Check sheet for the modelled part. Datum: model origin and axes. Units: mm. A direction names the side the tool comes from. Round coordinates to 2 decimals unless told otherwise and drop trailing zeros. Loops run counter-clockwise (first coordinate to the right, second up) from the corner with the lowest first, then second, coordinate; pieces in that order, holes last. Notation, with made-up numbers: (-26, -22.5) - (29, -22.5) arc R29 cw to (29, 5.5) - close; hole circle Ø8 at (74, 59.5). An arc over 180 degrees is marked (long way). Answer in a Markdown table with one row per item. Add a question column.
(1) Cross-section at D-D on y = 0. Enter the section's corners in (x, z).
(2) Gauge pin test, flat ends, axial feed: pin 1 (4.5 mm diameter, centred on y = -8.5, z = 7, fed in from -X); pin 2 (2 mm diameter, centred on y = 2.5, z = 9.5, fed in from +X); pin 3 (6 mm diameter, centred on y = -14.5, z = 7.5, fed in from +X); pin 4 (1.2 mm diameter, centred on x = -6.85, z = 8, fed in from -Y). Record the tip position at first contact, or that the pin passes through.
(3) Mould release check, pull along Y, two halves, no side actions. Record for faces 4 (the cylindrical face through (15.36, -19.19, 8.13)), 5 (the flat face through (0, 10, 3)), 6 (the cylindrical face through (4.608, 0.361, 4.056)): +Y half, -Y half, draft (parallel to the pull), parting line (faces both ways), or undercut.
(4) Cross-section at C-C on z = 3.25. Enter the section's corners in (x, y).
(5) Cross-section at B-B on x = -27.5. Enter the section's corners in (y, z), then the cut area to 3 significant figures.
(6) Access from +Z, -Z, +X, -X, +Y, -Y to the whole of each face (thin tool, end or side, straight path). Record for faces 1 (the flat face through (-5.5, 7, 6)), 2 (the flat face through (-21.6, -15, 6)), 3 (the flat face through (5.5, -8, 6)).
(7) Thickness scan on line 1 along Y through (x, z) = (-2, 5.25); line 2 along X through (y, z) = (-19.15, 8); line 3 along X through (y, z) = (-17.25, 2.75). Record the ranges inside material, lowest first.
(8) Cross-section at A-A on y = -17.75. Enter the section's corners in (x, z), then the cut area to 3 significant figures.
Autodesk Inventor part; units mm, degrees
ref_plane "YZ Plane" through (0, 0, 0) normal (1, 0, 0) x (0, 1, 0)
ref_plane "XZ Plane" through (0, 0, 0) normal (0, 1, 0) x (-1, 0, 0)
ref_plane "XY Plane" through (0, 0, 0) normal (0, 0, 1) x (1, 0, 0)
sketch "Эскиз1" plane through (0, 0, 0) normal (0, 0, 1) x (1, 0, 0)
  line L0 (-24, 10) -> (24, 10)
  line L1 (24, 10) -> (24, -10) construction
  line L2 (24, -10) -> (-24, -10)
  line L3 (-24, -10) -> (-24, 10) construction
  line L4 (0, 10) -> (0, -10)
  arc A0 (-30.4971, 2.649) -> (-30.4971, -2.649) centre (-27.5, 0) ccw
  line L5 (-30.4971, 2.649) -> (-24, 10)
  line L6 (-30.4971, -2.649) -> (-24, -10)
  arc A1 (30.4971, -2.649) -> (30.4971, 2.649) centre (27.5, 0) ccw
  line L7 (30.4971, 2.649) -> (24, 10)
  line L8 (30.4971, -2.649) -> (24, -10)
  point P0 (0, 0)
  point P1 (0, 0)
  dimension "d0" = 20
  dimension "d1" = 48
  dimension "d2" = 4
  dimension "d3" = 55
extrude "Выдавливание1" add sketch "Эскиз1" along normal blind 2
sketch "Эскиз2" plane through (0, 0, 2) normal (0, 0, 1) x (1, 0, 0)
  line L0 (24, 10) -> (-24, 10)
  line L1 (24, -10) -> (30.4971, -2.649)
  line L2 (-24, 10) -> (24, 10)
  line L3 (24, 10) -> (24, -10)
  line L4 (24, -10) -> (-24, -10)
  line L5 (-24, -10) -> (-24, 10)
  point P0 (0, 0)
extrude "Выдавливание2" add sketch "Эскиз2" along normal blind 6
sketch "Эскиз3" plane through (0, 0, 8) normal (0, 0, 1) x (1, 0, 0)
  circle A0 centre (-12.8, 0) radius 8.2
  circle A1 centre (12.8, 0) radius 8.2
  line L0 (-24, -10) -> (24, -10)
  line L1 (0, -10) -> (0, 10)
  line L2 (24, 10) -> (-24, 10)
  point P0 (0, 0)
  dimension "d8" = 25.6
  dimension "d9" = 16.4
extrude "Выдавливание3" cut sketch "Эскиз3" against normal through all
sketch "Эскиз4" plane through (0, 0, 8) normal (0, 0, 1) x (1, 0, 0)
  line L0 (24, 10) -> (-24, 10)
  line L1 (-5.5, 10) -> (5.5, 10)
  line L2 (5.5, 10) -> (5.5, 5)
  line L3 (5.5, 5) -> (-5.5, 5)
  line L4 (-5.5, 5) -> (-5.5, 10)
  line L5 (-24, 10) -> (-24, -10) construction
  line L6 (-24, 0) -> (24, 0)
  line L7 (24, -10) -> (24, 10) construction
  line L8 (-5.5, -10) -> (5.5, -10)
  line L9 (5.5, -10) -> (5.5, -5)
  line L10 (5.5, -5) -> (-5.5, -5)
  line L11 (-5.5, -5) -> (-5.5, -10)
  point P0 (0, 0)
  point P1 (0, 0)
  point P2 (0, 5)
  point P3 (0, -5)
  dimension "d12" = 5
  dimension "d13" = 11
extrude "Выдавливание4" cut sketch "Эскиз4" against normal blind 4
sketch "Эскиз5" plane through (0, 0, 2) normal (0, 0, 1) x (1, 0, 0)
  arc A0 (-30.4971, 2.649) -> (-30.4971, -2.649) centre (-27.5, 0) ccw
  arc A1 (30.4971, -2.649) -> (30.4971, 2.649) centre (27.5, 0) ccw
  point P0 (0, 0)
  point P1 (27.5, 0)
hole "Отверстие1" at (-27.5, 0, 2) at (27.5, 0, 2) direction (0, 0, -1) diameter 2.8 end through all
sketch "Эскиз6" plane through (0, 0, 0) normal (0, 0, -1) x (-1, 0, 0)
  line L0 (24, -10) -> (-24, -10)
  line L1 (24, -10) -> (-24, -10)
  line L2 (-24, -10) -> (-24, -20)
  line L3 (-24, -20) -> (24, -20)
  line L4 (24, -20) -> (24, -10)
  line L5 (-5.5, -10) -> (5.5, -10)
  line L6 (0, -20) -> (0, -10)
  line L7 (21.6, -18.4) -> (1.6, -18.4)
  line L8 (1.6, -18.4) -> (1.6, -11.4)
  line L9 (1.6, -11.4) -> (21.6, -11.4)
  line L10 (21.6, -11.4) -> (21.6, -18.4)
  line L11 (-1.6, -11.4) -> (-21.6, -11.4)
  line L12 (-21.6, -11.4) -> (-21.6, -18.4)
  line L13 (-21.6, -18.4) -> (-1.6, -18.4)
  line L14 (-1.6, -18.4) -> (-1.6, -11.4)
  point P0 (0, 0)
  point P1 (0, -10)
  dimension "d25" = 10
  dimension "d26" = 48
  dimension "d41" = 20
  dimension "d42" = 7
  dimension "d43" = 1.6
  dimension "d44" = 3.2
extrude "Выдавливание5" add sketch "Эскиз6" against normal blind 12
sketch "Эскиз7" plane through (-24, -20, 0) normal (0, -1, 0) x (1, 0, 0)
  line L0 (24, 0) -> (24, 12)
  line L1 (48, 0) -> (0, 0)
  line L2 (48, 0) -> (0, 0)
  line L3 (48, 0) -> (48, 12)
  line L4 (0, 12) -> (48, 12)
  line L5 (0, 0) -> (0, 12)
  line L6 (45.6, 0) -> (25.6, 0)
  line L7 (45.6, 0) -> (45.6, 12)
  line L8 (25.6, 12) -> (45.6, 12)
  line L9 (25.6, 0) -> (25.6, 12)
  line L10 (22.4, 0) -> (2.4, 0)
  line L11 (22.4, 0) -> (22.4, 12)
  line L12 (2.4, 12) -> (22.4, 12)
  line L13 (2.4, 0) -> (2.4, 12)
  line L14 (0, 12) -> (48, 12)
  line L15 (12.4, 12) -> (12.4, 0)
  line L16 (45, 0) -> (28.6, 0)
  line L17 (35.6, 0) -> (35.6, 12)
  point P0 (7.65, 8)
  point P1 (17.15, 8)
  point P2 (30.85, 8)
  point P3 (40.35, 8)
  dimension "d46" = 9.5
  dimension "d47" = 8
hole "Отверстие2" at (-16.35, -20, 8) at (-6.85, -20, 8) at (6.85, -20, 8) at (16.35, -20, 8) direction (0, 1, 0) diameter 2 depth 11
properties part number "FrontSensor"
Answers:
| question | item | result |
|---|---|---|
| 1 | outline | (-31.5, 0) - (-28.9, 0) - (-28.9, 2) - (-31.5, 2) - close; (-26.1, 0) - (-21, 0) - (-21, 8) - (-24, 8) - (-24, 2) - (-26.1, 2) - close; (-4.6, 0) - (4.6, 0) - (4.6, 8) - (-4.6, 8) - close; (21, 0) - (26.1, 0) - (26.1, 2) - (24, 2) - (24, 8) - (21, 8) - close; (28.9, 0) - (31.5, 0) - (31.5, 2) - (28.9, 2) - close |
| 2 | pin 1 | stops at x = -24 |
| 2 | pin 2 | passes through |
| 2 | pin 3 | stops at x = 24 |
| 2 | pin 4 | stops at y = -9 |
| 3 | face 4 | draft |
| 3 | face 5 | +Y half |
| 3 | face 6 | undercut |
| 4 | outline | (-24, -20) - (24, -20) - (24, 10) - (-24, 10) - close; hole (-21.6, -18.4) - (-1.6, -18.4) - (-1.6, -11.4) - (-21.6, -11.4) - close; hole circle Ø16.4 at (-12.8, 0); hole (1.6, -18.4) - (21.6, -18.4) - (21.6, -11.4) - (1.6, -11.4) - close; hole circle Ø16.4 at (12.8, 0) |
| 5 | outline | (-6.04, 0) - (-1.4, 0) - (-1.4, 2) - (-6.04, 2) - close; (1.4, 0) - (6.04, 0) - (6.04, 2) - (1.4, 2) - close |
| 5 | area | 18.6 mm^2 |
| 6 | face 1 | +Z, +Y |
| 6 | face 2 | +Z, -Z |
| 6 | face 3 | +Z |
| 7 | line 1 | y = -20 to -18.4, -11.4 to -10, -5 to 5 |
| 7 | line 2 | x = -24 to -17.35, -15.35 to -7.85, -5.85 to 5.85, 7.85 to 15.35, 17.35 to 24 |
| 7 | line 3 | x = -24 to -21.6, -1.6 to 1.6, 21.6 to 24 |
| 8 | outline | (-24, 0) - (-21.6, 0) - (-21.6, 12) - (-24, 12) - close; (-1.6, 0) - (1.6, 0) - (1.6, 12) - (-1.6, 12) - close; (21.6, 0) - (24, 0) - (24, 12) - (21.6, 12) - close |
| 8 | area | 96.0 mm^2 |
